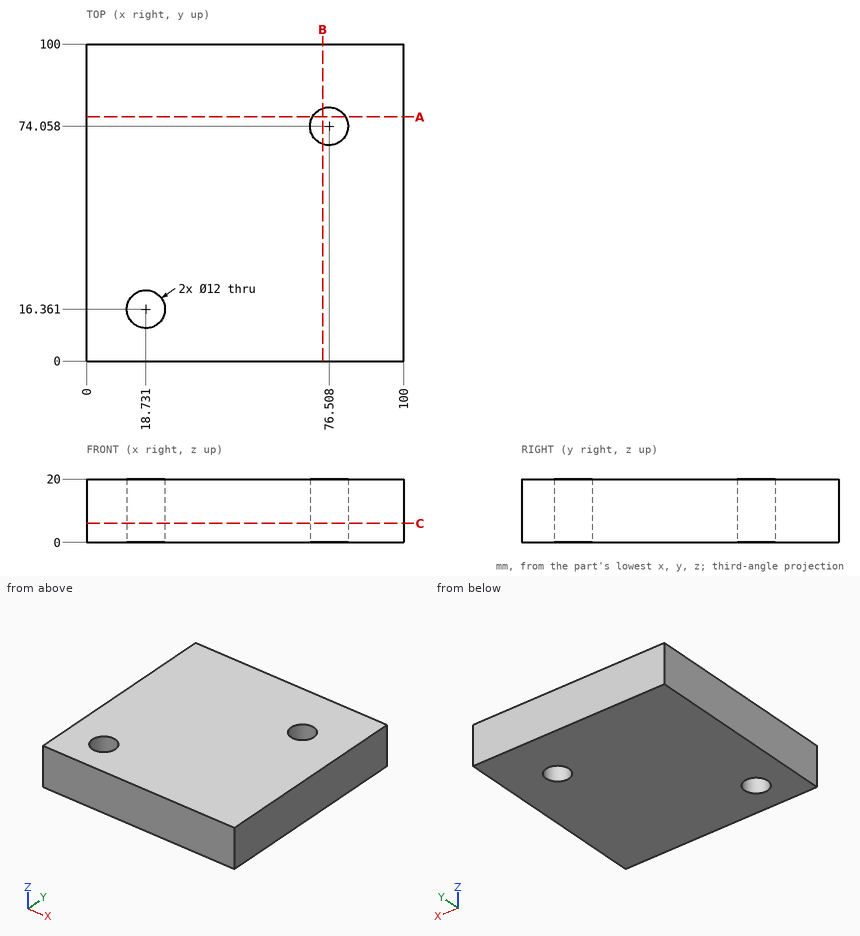
Geometry check sheet. Reference: drawing and pictorial views, mm from the part's lowest x, y, z. Coordinates: 2 decimals unless noted, no trailing zeros. Order: outer loops, then holes, each group sorted by start corner. A loop starts at its lowest first (then second) coordinate and runs counter-clockwise, first axis right, second up.
Item 1: Section check C-C (z = 6). Enter the section's corners in (x, y), plus the area to 3 significant figures.
Item 2: Section check A-A (y = 77). Enter the section's corners in (x, z).
Item 3: Section check B-B (x = 74.5). Enter the section's corners in (y, z).
Item 4: Scan lines: line 1 along Y through (x, z) = (76, 3.5); line 2 along X through (y, z) = (14.5, 9.25) (1 decimal); line 3 along Y through (x, z) = (80.5, 12.75). Record each from-to range of solid material in increasing order.
Item 5: Depth check by flat-ended pin: pin 1 (5 mm diameter, centred on y = 27, z = 14.5, fed in from -X). Enter the tip coordinate at first touch or a pass-through.
Check sheet entries:
1. outline: (0, 0) - (100, 0) - (100, 100) - (0, 100) - close; hole circle Ø12 at (18.73, 16.36); hole circle Ø12 at (76.51, 74.06)
1. area: 9,770 mm2
2. outline: (0, 0) - (71.28, 0) - (71.28, 20) - (0, 20) - close; (81.74, 0) - (100, 0) - (100, 20) - (81.74, 20) - close
3. outline: (0, 0) - (68.4, 0) - (68.4, 20) - (0, 20) - close; (79.71, 0) - (100, 0) - (100, 20) - (79.71, 20) - close
4. line 1: y = 0 to 68.08, 80.04 to 100
4. line 2: x = 0 to 13, 24.4 to 100
4. line 3: y = 0 to 69.58, 78.54 to 100
5. pin 1: stops at x = 0
